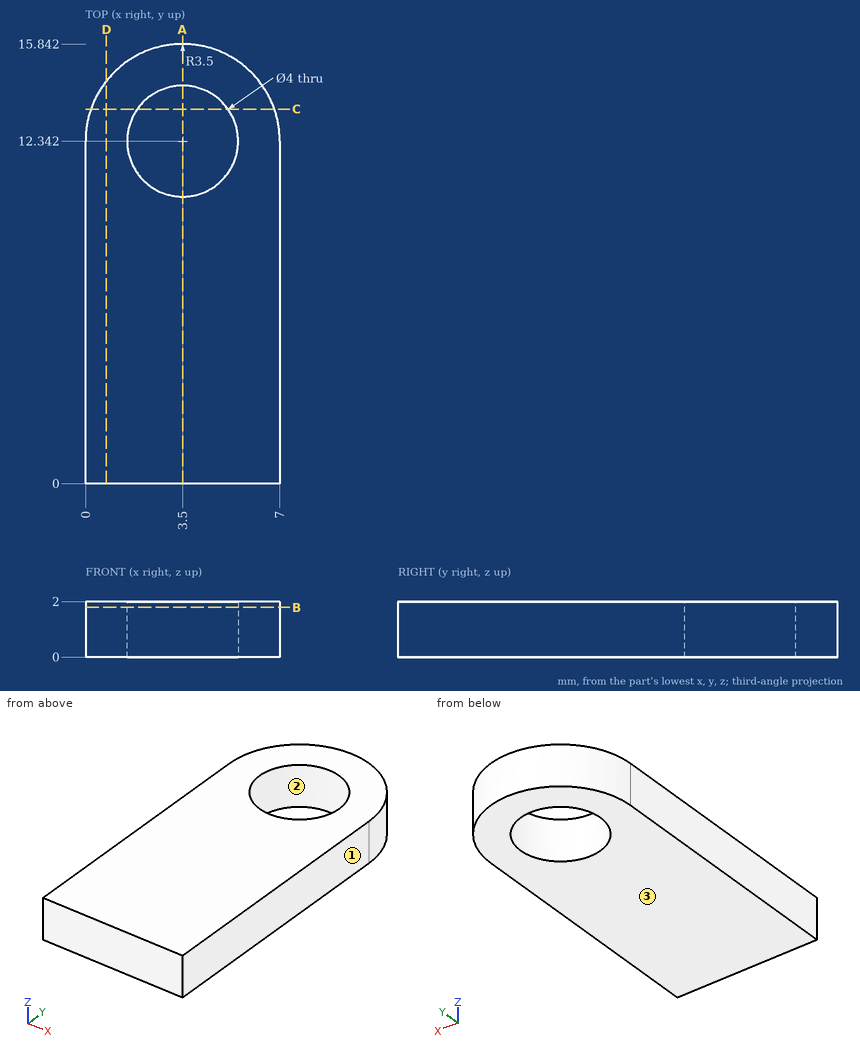
The drawing under review shows one solid part. Ordinate dimensions are in mm from its lowest x, y, z. Give positions to 0.01 mm unless a question says otherwise; leave off trailing zeros. Loops run counter-clockwise (first coordinate to the right, second up) from the corner with the lowest first, then second, coordinate; pieces in that order, holes last. Notation, with made-up numbers: M 20.25,75 L 26.25,75 A7 ccw 26.25,87 Z; hole C -5.5,-10.5 d6. An arc over 180 degrees is marked long. One line per item, written item: value. Start each with the question number.
Q1. Add section C-C (y = 13.5). Give the boundary of the cut face in (x, z).
Q2. For L1, parallel to Y at x = 3.5, z = 1; L2, parallel to Y at x = 3.75, z = 1.2; L3, parallel to X at y = 13, z = 0.7, list the stretches that pass through material, from the lowest coordinate up.
Q3. Add section A-A (x = 3.5). Give the boundary of the cut face in (y, z), and give its area (3 significant figures).
Q4. Draft analysis for pull direction X (two halves, no side actions). For the marked faces 1, 2 and 3, state which applies: released by +X, released by -X, zero draft, split by the parting line, or undercut.
Q5. Add section B-B (z = 1.8). Give the boundary of the cut face in (x, y).
Q6. Add section D-D (x = 0.75). Give the boundary of the cut face in (y, z), and give its area (3 significant figures).
Reply:
1. outline: M 0.2,0 L 1.87,0 L 1.87,2 L 0.2,2 Z; M 5.13,0 L 6.8,0 L 6.8,2 L 5.13,2 Z
2. L1: 0 to 10.34, 14.34 to 15.84
2. L2: 0 to 10.36, 14.33 to 15.83
2. L3: 0.06 to 1.61, 5.39 to 6.94
3. outline: M 0,0 L 10.34,0 L 10.34,2 L 0,2 Z; M 14.34,0 L 15.84,0 L 15.84,2 L 14.34,2 Z
3. area: 23.7 mm²
4. face 1: released by +X
4. face 2: undercut
4. face 3: zero draft
5. outline: M 0,0 L 7,0 L 7,12.34 A3.5 ccw 0,12.34 Z; hole C 3.5,12.34 d4
6. outline: M 0,0 L 14.51,0 L 14.51,2 L 0,2 Z
6. area: 29.0 mm²
